For this review, use the dimensioned drawing (mm, ordinates from the lowest corner) and the shaded views. A direction names the side the tool comes from. Coordinates: 2 decimals unless noted, no trailing zeros. Order: outer loops, then holes, each group sorted by start corner. A loop starts at its lowest first (then second) coordinate and runs counter-clockwise, first axis right, second up. Notation, with made-up numbers: M 71.5,-22 L 95.5,-22 A17 cw 95.5,-14 Z; hole C 78.5,38 d5. An arc over 180 degrees is marked long. Answer as CSV lines item,"result". Start each with the question number.
Q1. Machinability: for the marked faces 4, 5 and 6, which of the approach directions +Z, -Z, +X, -X, +Y, -Y give a long, thin tool a straight path to every point of the face, cutting with its end or side? Answer none if there is none.
Q2. Consider section C-C on x = 40.5. Write out the cut boundary in (y, z).
Q3. The part is to be moulded in two halves that separate along X. For the marked faces 1, 2 and 3, say which applies: +X half, -X half, draft (parallel to the pull), parting line (faces both ways), or undercut.
Q4. Wall thickness on L1, parallel to Y at x = 6, z = 5; L2, parallel to Z at x = 17.5, y = 9.5; L3, parallel to Y at x = 63.5, z = 33.5: over which ranges is each line inside the solid? List them lowest first. Write a range as [from, to].
Q5. Consider section B-B on z = 7.5. State how many separate pieces and enclosed holes the cut face has, and give its area (3 significant figures).
Q6. For P1, Ø5, axis at x = 43, z = 5, coming from the +Y side; P2, Ø5.5, axis at x = 66, z = 72.5, coming from the -Y side; P3, Ø5, axis at x = 44.5, y = 5.5, coming from the +Z side, all flat-tipped, find the tip position at first contact; note any pin that passes through.
Q7. Consider section D-D on y = 9.75. Write out the cut boundary in (x, z), and give its area (3 significant figures).
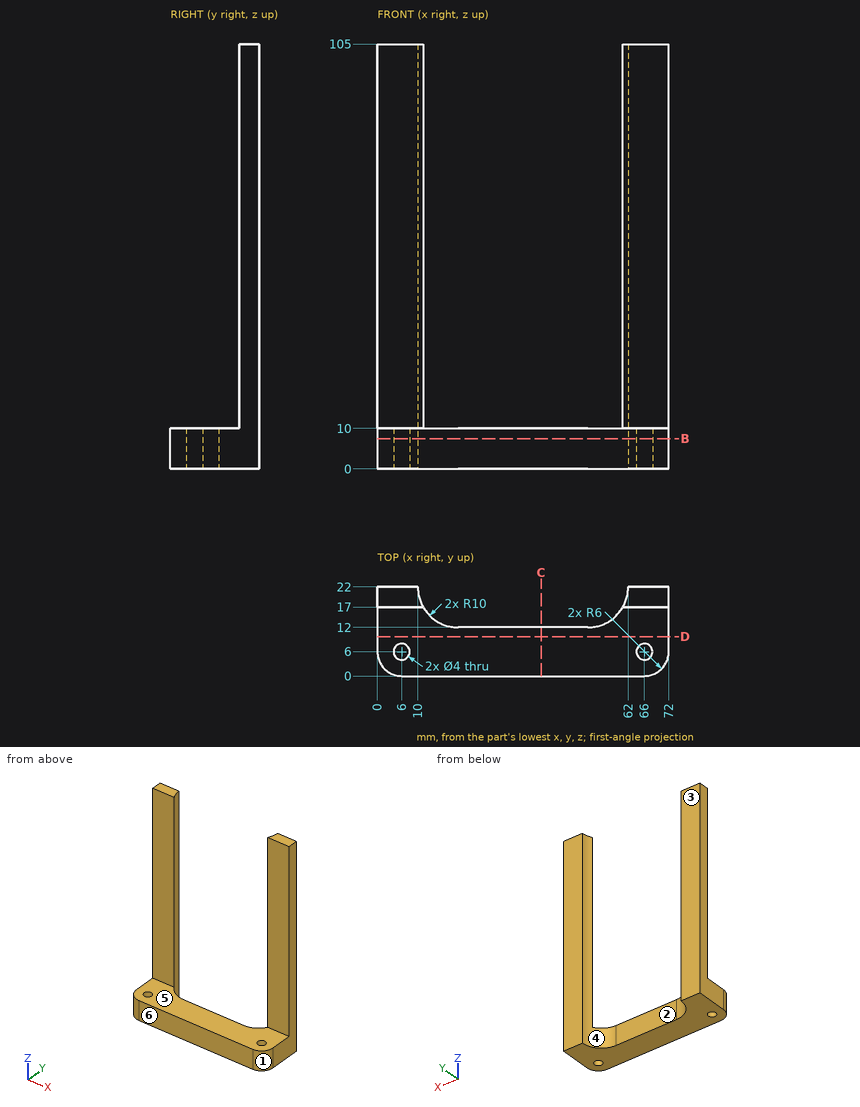
Evaluation:
1,face 4,"+Z, -Z, +Y"
1,face 5,"+Z, +X, -X, -Y"
1,face 6,"+Z, -Z, +X, -X, -Y"
2,outline,"M 0,0 L 12,0 L 12,10 L 0,10 Z"
3,face 1,"+X half"
3,face 2,"undercut"
3,face 3,"draft"
4,L1,"y = [0, 4], [8, 22]"
4,L2,"z = [0, 10]"
4,L3,"y = [17, 22]"
5,separate pieces,"1"
5,enclosed holes,"2"
5,area,"1,070 mm²"
6,P1,"stops at y = 12"
6,P2,"stops at y = 17"
6,P3,"stops at z = 10"
7,outline,"M 0,0 L 72,0 L 72,10 L 0,10 Z"
7,area,"720 mm²"
